The model under review builds one solid part; all positions refer to its coordinate system, in mm. Face numbers are marked on the shaded views. A direction names the side the tool comes from. Round coordinates to 2 decimals unless told otherwise and drop trailing zeros. Write each loop counter-clockwise with the first axis right and the second up, starting at its lowest first coordinate (ties: lowest second). Pieces come first, ordered by that corner, then holes. Notation, with made-up numbers: (-38.75, 78) -> (7.25, 78) arc R19 cw to (7.25, 82) -> close; hole circle Ø4 at (32.25, -29). An arc over 180 degrees is marked (long way). Use CSV: the item, a comma, the result in double quotes. Start each with the question number.
1) Mouldability with a two-part tool opening along X and no side actions: class the marked faces 1, 2 and 3 as released by +X, released by -X, zero draft, split by the parting line, or undercut.
2) Wall thickness on probe 1 along X at (y, z) = (20, 0); probe 2 along Y at (x, z) = (12, 0); probe 3 along Z at (x, y) = (0, 28.5): over which ranges is each line inside the solid? List them lowest first. Write a range as [from, to].
3) Take a section at B-B, the plane x = 7.75. Give the boundary of the cut face in (y, z) (1 decimal), then the cut area to 3 significant figures.
4) Machinability: for the marked faces 4 and 5, which of the approach directions +Z, -Z, +X, -X, +Y, -Y give a long, thin tool a straight path to every point of the face, cutting with its end or side? Answer none if there is none.
5) Take a section at C-C, the plane z = 0. Give the boundary of the cut face in (x, y), then the cut area to 3 significant figures.
6) Take a section at A-A, the plane y = 37. Give the boundary of the cut face in (x, z) (1 decimal).
7) For pin 1 Ø1 at (x, z) = (11, -2.5) entering from -Y; pin 2 Ø1.5 at (x, y) = (1, 13.5) entering from +Z; pin 3 Ø2 at (x, y) = (5, 28.5) entering from -Z; pin 4 Ø2 at (y, z) = (32, -1) entering from -X, all flat-tipped, find the tip position at first contact; note any pin that passes through.
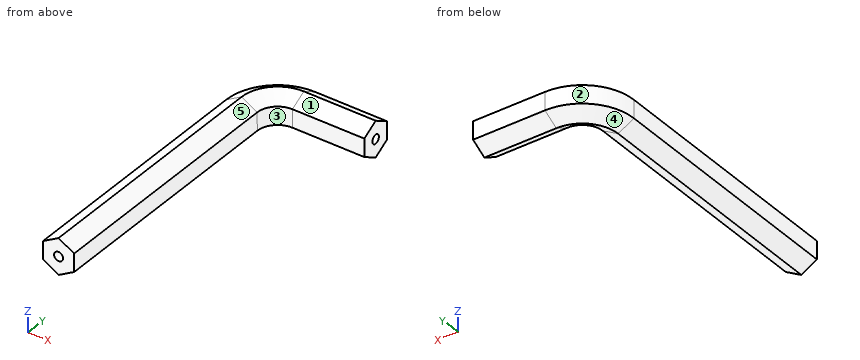
from build123d import *

# Parameters (mm, degrees)
F3_R = 0.79375


with BuildPart() as f2:
    # F2: sweep along a path in F1
    with BuildLine(Plane.XY) as f2_path:
        Line((0, 0), (0, 44.45))
        ThreePointArc((0, 44.45), (1.8598719395, 48.9401280605), (6.35, 50.8))
        Line((6.35, 50.8), (19.05, 50.8))
    # F0 (on Front) → F2 (sweep)
    with BuildSketch(Plane.XZ):
        Polygon((0.0141373198, -3.175), (2.7566993169, -1.5752567219), (2.7425619971, 1.5997432781), (-0.0141373198, 3.175), (-2.7566993169, 1.5752567219), (-2.7425619971, -1.5997432781), align=None)
    sweep(path=f2_path.line)

    # F4: sweep along a path in F1
    with BuildLine(Plane.XY) as f4_path:
        Line((0, 0), (0, 44.45))
        ThreePointArc((0, 44.45), (1.8598719395, 48.9401280605), (6.35, 50.8))
        Line((6.35, 50.8), (19.05, 50.8))
    # F3 (on Front) → F4 (sweep, cut)
    with BuildSketch(Plane.XZ):
        Circle(F3_R)
    sweep(path=f4_path.line, mode=Mode.SUBTRACT)


solid = f2.part
Values found:
1,face 1,"zero draft"
1,face 2,"released by -X"
1,face 3,"released by +X"
2,probe 1,"[-2.75, -0.79], [0.79, 2.75]"
2,probe 2,"[48.05, 50.01], [51.59, 53.55]"
2,probe 3,"[-3.17, -0.79], [0.79, 3.17]"
3,outline,"(48, -1.6) -> (50.8, -3.2) -> (53.5, -1.6) -> (53.6, 1.6) -> (50.8, 3.2) -> (48.1, 1.6) -> close; hole circle Ø1.6 at (50.8, 0)"
3,area,"24.2 mm²"
4,face 4,"-Z, -X, +Y"
4,face 5,"+Z, +X, -Y"
5,outline,"(-2.75, 0) -> (-0.79, 0) -> (-0.79, 44.45) arc R7.14 cw to (6.35, 51.59) -> (19.05, 51.59) -> (19.05, 53.55) -> (6.35, 53.55) arc R9.1 ccw to (-2.75, 44.45) -> close; (0.79, 0) -> (2.75, 0) -> (2.75, 44.45) arc R3.6 cw to (6.35, 48.05) -> (19.05, 48.05) -> (19.05, 50.01) -> (6.35, 50.01) arc R5.56 ccw to (0.79, 44.45) -> close"
5,area,"263 mm²"
6,outline,"(-2.8, 1.6) -> (-2.7, -1.6) -> (0, -3.2) -> (2.8, -1.6) -> (2.7, 1.6) -> (0, 3.2) -> close; hole circle Ø1.6 at (0, 0)"
7,pin 1,"y = 48.77"
7,pin 2,"z = 3.02"
7,pin 3,"through"
7,pin 4,"x = -2.75"
